Check sheet for the modelled part. Datum: model origin and axes. Units: mm. A direction names the side the tool comes from. Give positions to 0.01 mm unless a question says otherwise; leave off trailing zeros. Write each loop counter-clockwise with the first axis right and the second up, starting at its lowest first coordinate (ties: lowest second). Pieces come first, ordered by that corner, then holes.
from build123d import *

# Parameters (mm, degrees)
F1_DEPTH       = 25
F2_DEPTH       = 35
F3_DEPTH       = 55
F4_DEPTH       = 20
F5_SIZE2       = 5
F5_SIZE        = 5
F7_D           = 14.75
F7_CBORE_D     = 22.25
F7_CBORE_DEPTH = 14
F8_R           = 7.4840620434


with BuildPart() as f1:
    # F0 (on Front) → F1 (new body)
    with BuildSketch(Plane.XZ):
        with BuildLine():
            Line((106.5, -40), (106.5, 55))
            Line((106.5, 55), (48.7497216032, 55))
            ThreePointArc((48.7497216032, 55), (42.4942891815, 52.8018949761), (38.9888762464, 47.1739130435))
            ThreePointArc((38.9888762464, 47.1739130435), (10.7462120246, -4.2462120246), (-40.6739130435, -32.4888762464))
            ThreePointArc((-40.6739130435, -32.4888762464), (-46.3018949761, -35.9942891815), (-48.5, -42.2497216032))
            Line((-48.5, -42.2497216032), (-48.5, -100))
            Line((-48.5, -100), (46.5, -100))
            Line((46.5, -100), (46.5, -55))
            ThreePointArc((46.5, -55), (50.8933982822, -44.3933982822), (61.5, -40))
            Line((61.5, -40), (106.5, -40))
        make_face()
        with BuildLine():
            ThreePointArc((-29.5, -91), (-36.5710678119, -88.0710678119), (-39.5, -81))
            Line((-39.5, -81), (-39.5, -49.2476414861))
            ThreePointArc((-39.5, -49.2476414861), (-37.481834214, -43.2234965193), (-32.2419354839, -39.630896205))
            ThreePointArc((-32.2419354839, -39.630896205), (17.1101730553, -10.6101730553), (46.130896205, 38.7419354839))
            ThreePointArc((46.130896205, 38.7419354839), (49.7234965193, 43.981834214), (55.7476414861, 46))
            Line((55.7476414861, 46), (87.5, 46))
            ThreePointArc((87.5, 46), (94.5710678119, 43.0710678119), (97.5, 36))
            Line((97.5, 36), (97.5, -21))
            ThreePointArc((97.5, -21), (94.5710678119, -28.0710678119), (87.5, -31))
            Line((87.5, -31), (61.5, -31))
            ThreePointArc((61.5, -31), (44.5294372515, -38.0294372515), (37.5, -55))
            Line((37.5, -55), (37.5, -81))
            ThreePointArc((37.5, -81), (34.5710678119, -88.0710678119), (27.5, -91))
            Line((27.5, -91), (-29.5, -91))
        make_face(mode=Mode.SUBTRACT)
        with BuildLine():
            Line((96.5, 100), (-96.5, 100))
            ThreePointArc((-96.5, 100), (-103.5710678119, 97.0710678119), (-106.5, 90))
            Line((-106.5, 90), (-106.5, -90))
            ThreePointArc((-106.5, -90), (-103.5710678119, -97.0710678119), (-96.5, -100))
            Line((-96.5, -100), (-63.5, -100))
            Line((-63.5, -100), (-63.5, -42.2497216032))
            ThreePointArc((-63.5, -42.2497216032), (-58.0047374401, -26.6111405489), (-43.9347826087, -17.8476082112))
            ThreePointArc((-43.9347826087, -17.8476082112), (0.1396103068, 6.3603896932), (24.3476082112, 50.4347826087))
            ThreePointArc((24.3476082112, 50.4347826087), (33.1111405489, 64.5047374401), (48.7497216032, 70))
            Line((48.7497216032, 70), (106.5, 70))
            Line((106.5, 70), (106.5, 90))
            ThreePointArc((106.5, 90), (103.5710678119, 97.0710678119), (96.5, 100))
        make_face()
        with BuildLine():
            ThreePointArc((14.7304288624, 91), (-11.3221396288, 8.044605666), (-97.5, -3.5187051029))
            Line((-97.5, -3.5187051029), (-97.5, 91))
            Line((-97.5, 91), (14.7304288624, 91))
        make_face(mode=Mode.SUBTRACT)
        with BuildLine():
            Line((-97.5, 91), (-97.5, -3.5187051029))
            ThreePointArc((-97.5, -3.5187051029), (-11.3221396288, 8.044605666), (14.7304288624, 91))
            Line((14.7304288624, 91), (-97.5, 91))
        make_face()
        with BuildLine():
            Line((-39.5, -49.2476414861), (-39.5, -81))
            ThreePointArc((-39.5, -81), (-36.5710678119, -88.0710678119), (-29.5, -91))
            Line((-29.5, -91), (27.5, -91))
            ThreePointArc((27.5, -91), (34.5710678119, -88.0710678119), (37.5, -81))
            Line((37.5, -81), (37.5, -55))
            ThreePointArc((37.5, -55), (44.5294372515, -38.0294372515), (61.5, -31))
            Line((61.5, -31), (87.5, -31))
            ThreePointArc((87.5, -31), (94.5710678119, -28.0710678119), (97.5, -21))
            Line((97.5, -21), (97.5, 36))
            ThreePointArc((97.5, 36), (94.5710678119, 43.0710678119), (87.5, 46))
            Line((87.5, 46), (55.7476414861, 46))
            ThreePointArc((55.7476414861, 46), (49.7234965193, 43.981834214), (46.130896205, 38.7419354839))
            ThreePointArc((46.130896205, 38.7419354839), (17.1101730553, -10.6101730553), (-32.2419354839, -39.630896205))
            ThreePointArc((-32.2419354839, -39.630896205), (-37.481834214, -43.2234965193), (-39.5, -49.2476414861))
        make_face()
        with BuildLine():
            Line((106.5, 55), (106.5, 70))
            Line((106.5, 70), (48.7497216032, 70))
            ThreePointArc((48.7497216032, 70), (33.1111405489, 64.5047374401), (24.3476082112, 50.4347826087))
            ThreePointArc((24.3476082112, 50.4347826087), (0.1396103068, 6.3603896932), (-43.9347826087, -17.8476082112))
            ThreePointArc((-43.9347826087, -17.8476082112), (-58.0047374401, -26.6111405489), (-63.5, -42.2497216032))
            Line((-63.5, -42.2497216032), (-63.5, -100))
            Line((-63.5, -100), (-48.5, -100))
            Line((-48.5, -100), (-48.5, -42.2497216032))
            ThreePointArc((-48.5, -42.2497216032), (-46.3018949761, -35.9942891815), (-40.6739130435, -32.4888762464))
            ThreePointArc((-40.6739130435, -32.4888762464), (10.7462120246, -4.2462120246), (38.9888762464, 47.1739130435))
            ThreePointArc((38.9888762464, 47.1739130435), (42.4942891815, 52.8018949761), (48.7497216032, 55))
            Line((48.7497216032, 55), (106.5, 55))
        make_face()
        with BuildLine():
            Line((106.5, -90), (106.5, -40))
            Line((106.5, -40), (61.5, -40))
            ThreePointArc((61.5, -40), (50.8933982822, -44.3933982822), (46.5, -55))
            Line((46.5, -55), (46.5, -100))
            Line((46.5, -100), (96.5, -100))
            ThreePointArc((96.5, -100), (103.5710678119, -97.0710678119), (106.5, -90))
        make_face()
    extrude(amount=-F1_DEPTH)

    # F0 (on Front) → F2 (join)
    with BuildSketch(Plane.XZ):
        with BuildLine():
            Line((-97.5, 91), (-97.5, -3.5187051029))
            ThreePointArc((-97.5, -3.5187051029), (-11.3221396288, 8.044605666), (14.7304288624, 91))
            Line((14.7304288624, 91), (-97.5, 91))
        make_face()
        with BuildLine():
            Line((106.5, -90), (106.5, -40))
            Line((106.5, -40), (61.5, -40))
            ThreePointArc((61.5, -40), (50.8933982822, -44.3933982822), (46.5, -55))
            Line((46.5, -55), (46.5, -100))
            Line((46.5, -100), (96.5, -100))
            ThreePointArc((96.5, -100), (103.5710678119, -97.0710678119), (106.5, -90))
        make_face()
    extrude(amount=F2_DEPTH)

    # F0 (on Front) → F3 (join)
    with BuildSketch(Plane.XZ):
        with BuildLine():
            Line((106.5, 55), (106.5, 70))
            Line((106.5, 70), (48.7497216032, 70))
            ThreePointArc((48.7497216032, 70), (33.1111405489, 64.5047374401), (24.3476082112, 50.4347826087))
            ThreePointArc((24.3476082112, 50.4347826087), (0.1396103068, 6.3603896932), (-43.9347826087, -17.8476082112))
            ThreePointArc((-43.9347826087, -17.8476082112), (-58.0047374401, -26.6111405489), (-63.5, -42.2497216032))
            Line((-63.5, -42.2497216032), (-63.5, -100))
            Line((-63.5, -100), (-48.5, -100))
            Line((-48.5, -100), (-48.5, -42.2497216032))
            ThreePointArc((-48.5, -42.2497216032), (-46.3018949761, -35.9942891815), (-40.6739130435, -32.4888762464))
            ThreePointArc((-40.6739130435, -32.4888762464), (10.7462120246, -4.2462120246), (38.9888762464, 47.1739130435))
            ThreePointArc((38.9888762464, 47.1739130435), (42.4942891815, 52.8018949761), (48.7497216032, 55))
            Line((48.7497216032, 55), (106.5, 55))
        make_face()
    extrude(amount=F3_DEPTH)

    # F0 (on Front) → F4 (cut)
    with BuildSketch(Plane.XZ):
        with BuildLine():
            Line((-39.5, -49.2476414861), (-39.5, -81))
            ThreePointArc((-39.5, -81), (-36.5710678119, -88.0710678119), (-29.5, -91))
            Line((-29.5, -91), (27.5, -91))
            ThreePointArc((27.5, -91), (34.5710678119, -88.0710678119), (37.5, -81))
            Line((37.5, -81), (37.5, -55))
            ThreePointArc((37.5, -55), (44.5294372515, -38.0294372515), (61.5, -31))
            Line((61.5, -31), (87.5, -31))
            ThreePointArc((87.5, -31), (94.5710678119, -28.0710678119), (97.5, -21))
            Line((97.5, -21), (97.5, 36))
            ThreePointArc((97.5, 36), (94.5710678119, 43.0710678119), (87.5, 46))
            Line((87.5, 46), (55.7476414861, 46))
            ThreePointArc((55.7476414861, 46), (49.7234965193, 43.981834214), (46.130896205, 38.7419354839))
            ThreePointArc((46.130896205, 38.7419354839), (17.1101730553, -10.6101730553), (-32.2419354839, -39.630896205))
            ThreePointArc((-32.2419354839, -39.630896205), (-37.481834214, -43.2234965193), (-39.5, -49.2476414861))
        make_face()
    extrude(amount=-F4_DEPTH, mode=Mode.SUBTRACT)

    # F5
    f5_edges = [f1.edges().sort_by_distance(p)[0] for p in [
        (-11.32214, -35, 8.044606),
        (-41.384786, -35, 91),
        (-97.5, -35, 43.740647),
    ]]
    chamfer(f5_edges, length=F5_SIZE, length2=F5_SIZE2)

    # F7 (through all)
    with Locations(Plane.XZ.offset(35)):
        with Locations((76.5, -70)):
            CounterBoreHole(F7_D / 2, F7_CBORE_D / 2, F7_CBORE_DEPTH)

    # F8
    f8_edges = [f1.edges().sort_by_distance(p)[0] for p in [
        (-48.5, -55, -71.124861),
        (-63.5, -55, -71.124861),
    ]]
    fillet(f8_edges, radius=F8_R)


solid = f1.part
1) Draft check along X on faces 4 (the cylindrical face through (77.221, -52.749, 67.866)), 5 (the cylindrical face through (-61.366, -52.749, -71.529)), 6 (the flat face through (40, 0, -45)). Enter one of: +X half, -X half, draft (parallel to the pull), parting line (faces both ways), or undercut.
2) Gauge pin test, flat ends, axial feed: pin 1 (24.5 mm diameter, centred on x = 74, z = -70.5, fed in from -Y); pin 2 (1.5 mm diameter, centred on x = 61.5, y = -39.5, fed in from -Z); pin 3 (4 mm diameter, centred on x = -27, z = -64.5, fed in from -Y). Record the tip position at first contact, or that the pin passes through.
3) Sectioned sample at C-C on x = 76.5. Record the boundary of the cut face in (y, z) (3 decimals).
4) Access from +Z, -Z, +X, -X, +Y, -Y to the whole of each face (thin tool, end or side, straight path). Record for faces 1 (the cylindrical face through (-46.36, -23.43, -36.07)), 2 (the cylindrical face through (51.01, -17.26, -44.28)), 3 (the flat face through (-97.5, -15, 44)).
5) Sectioned sample at B-B on z = -70. Record the boundary of the cut face in (x, y) (3 decimals), then the cut area to 3 significant figures.
6) Sectioned sample at A-A on y = -3. Record the boundary of the cut face in (x, z) (3 decimals).
7) Scan lines: L1, parallel to X at y = -5.5, z = -70.5; L2, parallel to Z at x = 76.5, y = -30.75 (3 decimals); L3, parallel to Z at x = 76.5, y = 5.5 (3 decimals). Record each from-to range of solid material in increasing order.
Answers below:
1. face 4: draft
1. face 5: -X half
1. face 6: undercut
2. pin 1: stops at y = -35
2. pin 2: stops at z = 55
2. pin 3: stops at y = 20
3. outline: (-55, 62.484) arc R7.484 ccw to (-47.516, 55) - (0, 55) - (0, 46) - (20, 46) - (20, -31) - (0, -31) - (0, -40) - (-35, -40) - (-35, -58.875) - (-21, -58.875) - (-21, -62.625) - (25, -62.625) - (25, 100) - (0, 100) - (0, 70) - (-47.516, 70) arc R7.484 ccw to (-55, 62.516) - close; (-35, -100) - (25, -100) - (25, -77.375) - (-21, -77.375) - (-21, -81.125) - (-35, -81.125) - close
4. face 1: -Z, -Y
4. face 2: -Y
4. face 3: +Z, -Z, -X, -Y
5. outline: (-106.5, 0) - (-63.5, 0) - (-63.5, -47.516) arc R7.484 ccw to (-56.016, -55) - (-55.984, -55) arc R7.484 ccw to (-48.5, -47.516) - (-48.5, 0) - (-39.5, 0) - (-39.5, 20) - (37.5, 20) - (37.5, 0) - (46.5, 0) - (46.5, -35) - (65.375, -35) - (65.375, -21) - (69.125, -21) - (69.125, 25) - (-106.5, 25) - close; (83.875, -21) - (87.625, -21) - (87.625, -35) - (106.5, -35) - (106.5, 25) - (83.875, 25) - close
5. area: 5,700 mm2
6. outline: (-97.5, -3.519) arc R81 ccw to (14.73, 91) - (-97.5, 91) - close; (-63.5, -100) - (-48.5, -100) - (-48.5, -42.25) arc R10 cw to (-40.674, -32.489) arc R105 ccw to (38.989, 47.174) arc R10 cw to (48.75, 55) - (106.5, 55) - (106.5, 70) - (48.75, 70) arc R25 ccw to (24.348, 50.435) arc R90 cw to (-43.935, -17.848) arc R25 ccw to (-63.5, -42.25) - close; (46.5, -100) - (96.5, -100) arc R10 ccw to (106.5, -90) - (106.5, -40) - (61.5, -40) arc R15 ccw to (46.5, -55) - close; hole circle Ø14.75 at (76.5, -70)
7. L1: x = -63.5 to -48.5, 46.5 to 69.14, 83.86 to 106.5
7. L2: z = -100 to -81.125, -58.875 to -40, 55 to 70
7. L3: z = -100 to -77.375, -62.625 to -31, 46 to 100
